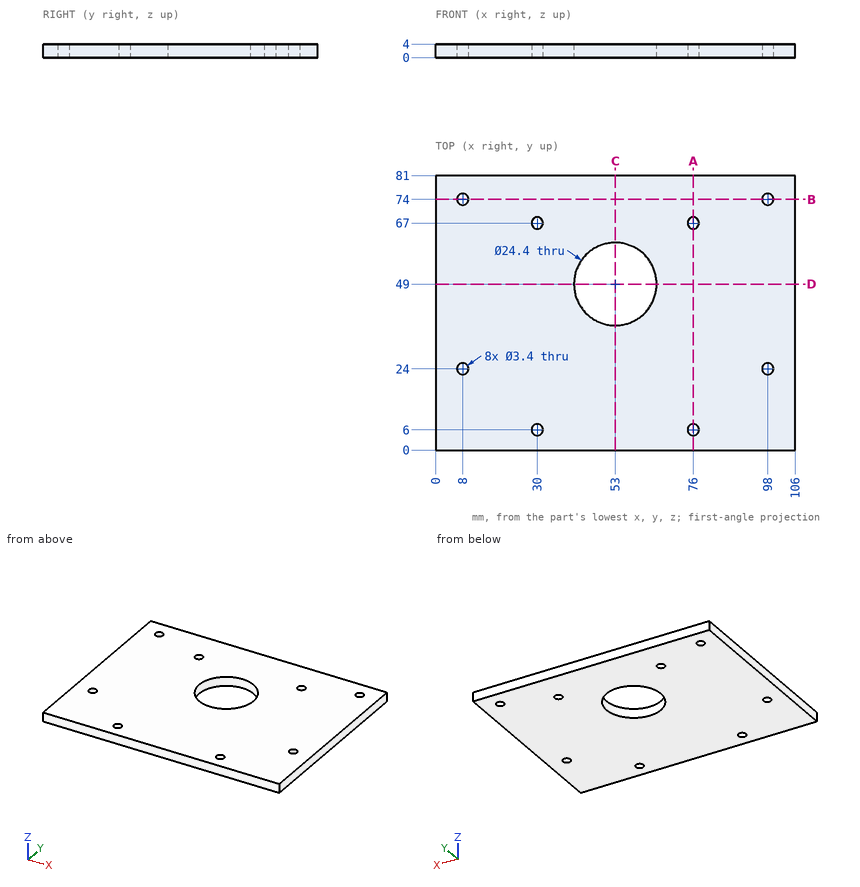
Print and shaded views of the part. All mm, measured from the part's lowest x, y and z. Coordinates: 2 decimals unless noted, no trailing zeros. Order: outer loops, then holes, each group sorted by start corner. A loop starts at its lowest first (then second) coordinate and runs counter-clockwise, first axis right, second up. Notation, with made-up numbers: M 74,80 L 93,80 A23 cw 93,101 Z; hole C 79,48.5 d10. An arc over 180 degrees is marked long. Write each question's results on one line, items separated by ' | '. Start each with the question number.
Q1. Drill centre lines: probe 1 along Y at (x, z) = (76, 2.5); probe 2 along Y at (x, z) = (98, 2.7); probe 3 along X at (y, z) = (74, 2.65). Where is each one in solid material? Low to high. Write a range as from..to.
Q2. Cut at A-A (x = 76). List the corners of the cut face in (y, z).
Q3. Cut at C-C (x = 53). List the corners of the cut face in (y, z).
Q4. Cut at B-B (y = 74). List the corners of the cut face in (x, z).
Q5. Cut at D-D (y = 49). List the corners of the cut face in (x, z).
Found:
1) probe 1: 0..4.3, 7.7..65.3, 68.7..81 | probe 2: 0..22.3, 25.7..72.3, 75.7..81 | probe 3: 0..6.3, 9.7..96.3, 99.7..106
2) outline: M 0,0 L 4.3,0 L 4.3,4 L 0,4 Z; M 7.7,0 L 65.3,0 L 65.3,4 L 7.7,4 Z; M 68.7,0 L 81,0 L 81,4 L 68.7,4 Z
3) outline: M 0,0 L 36.8,0 L 36.8,4 L 0,4 Z; M 61.2,0 L 81,0 L 81,4 L 61.2,4 Z
4) outline: M 0,0 L 6.3,0 L 6.3,4 L 0,4 Z; M 9.7,0 L 96.3,0 L 96.3,4 L 9.7,4 Z; M 99.7,0 L 106,0 L 106,4 L 99.7,4 Z
5) outline: M 0,0 L 40.8,0 L 40.8,4 L 0,4 Z; M 65.2,0 L 106,0 L 106,4 L 65.2,4 Z
